Verification items for the finished model (mm, model axes). Give positions to 0.01 mm unless a question says otherwise; leave off trailing zeros. Loops run counter-clockwise (first coordinate to the right, second up) from the corner with the lowest first, then second, coordinate; pieces in that order, holes last. Notation, with made-up numbers: (-28, 11) - (-3, 11) arc R22 cw to (-3, 39) - close; hole circle Ø8 at (-28, -0.5). An arc over 180 degrees is marked (long way). Answer in a Markdown table with one row per item.
```python
from build123d import *

# Parameters (mm, degrees)
SKETCH1_R             = 2.625
BOSS_EXTRUDE1_DEPTH   = 4
FILLET1_R             = 35
FILLET2_R             = 8
SKETCH2_R             = 5.05
CUT_EXTRUDE1_DEPTH    = 1
FILLET3_R             = 1
FILLET7_R             = 4
MIRROR1_OUTLINE_R     = 5.05
MIRROR1_DEPTH         = 4
MIRROR1_2_OUTLINE_R   = 5.05
MIRROR1_2_OUTLINE_R_2 = 2.625
MIRROR1_2_DEPTH       = 3
FILLET6_R             = 1
SKETCH3_R             = 6
BOSS_EXTRUDE2_DEPTH   = 4
FILLET8_R             = 4


with BuildPart() as part:
    # Sketch1 → Boss-Extrude1 (new body)
    with BuildSketch(Plane(origin=(0, 0, 0), x_dir=(1, 0, 0), z_dir=(0, 1, 0))):
        with BuildLine():
            Line((-0.828427125, -40), (15.171572875, -40))
            ThreePointArc((15.171572875, -40), (16.585786438, -39.414213562), (17.171572875, -38))
            Line((17.171572875, -38), (17.171572875, -10.175438596))
            Line((17.171572875, -10.175438596), (17.171572875, 18))
            ThreePointArc((17.171572875, 18), (16.585786438, 19.414213562), (15.171572875, 20))
            Line((15.171572875, 20), (-40.828427125, 20))
            ThreePointArc((-40.828427125, 20), (-42.242640687, 19.414213562), (-42.828427125, 18))
            Line((-42.828427125, 18), (-42.828427125, 2))
            Line((-42.828427125, 2), (-42.828427125, -4))
            Line((-42.828427125, -4), (-6.828427125, -40))
            Line((-6.828427125, -40), (-0.828427125, -40))
        make_face()
        with Locations(Location((-32.828427125, 10, 0), (0, 0, 270))):
            Circle(SKETCH1_R, mode=Mode.SUBTRACT)
        with Locations(Location((-12.828427125, 10, 0), (0, 0, 270))):
            Circle(SKETCH1_R, mode=Mode.SUBTRACT)
        with Locations(Location((7.171572875, -32, 0), (0, 0, 270))):
            Circle(SKETCH1_R, mode=Mode.SUBTRACT)
        with Locations(Location((7.171572875, 10, 0), (0, 0, 270))):
            Circle(SKETCH1_R, mode=Mode.SUBTRACT)
        with Locations(Location((7.171572875, -11, 0), (0, 0, 270))):
            Circle(SKETCH1_R, mode=Mode.SUBTRACT)
        Polygon((0, 0), (0, -34.343145751), (-4, -34.343145751), (-34.343145751, -4), (-34.343145751, 0), align=None, mode=Mode.SUBTRACT)
    extrude(amount=BOSS_EXTRUDE1_DEPTH)

    # Fillet1
    # the kernel refuses this fillet: 35 mm, written as the material it adds along each edge
    with BuildSketch(Plane(origin=(0, 0, 0), x_dir=(-1, 0, 0), z_dir=(0, 1, 0))) as fillet1_piece_1:
        with BuildLine():
            CenterArc((34.993835779, 35), FILLET1_R, 181.075348167, 88.924651833)
            Line((0, 34.343145751), (-0.699876716, 34.330008666))
            ThreePointArc((-0.699876716, 34.330008666), (-0.7, 17.171572875), (-0.7, 0))
            Line((-0.7, 0), (0, -0.7))
            Line((0, -0.7), (34.993835779, -0.7))
            Line((34.993835779, -0.7), (34.993835779, 0))
        make_face()
    extrude(amount=4)

    # Fillet2
    # the kernel refuses this fillet: 8 mm, written as the material it adds along each edge
    with BuildSketch(Plane(origin=(0, 0, 34.343145751), x_dir=(-0.13953759415061998, 0, -0.9902167741553647), z_dir=(0, 1, 0))) as fillet2_piece_1:
        with BuildLine():
            CenterArc((7.497620247, 7.941288924), FILLET2_R, 209.838221464, 67.107520075)
            Line((0.558150377, 3.960867097), (0, 0))
            ThreePointArc((0, 0), (4.232527559, -0.256860958), (8.465055117, 0))
        make_face()
    extrude(amount=4)
    with BuildSketch(Plane(origin=(-34.343145751, 4, 0.006049059), x_dir=(0.9902532983948017, 0, 0.13927815700322774), z_dir=(0, -1, 0))) as fillet2_piece_2:
        with BuildLine():
            CenterArc((7.49233694, 7.941371943), FILLET2_R, 209.887169965, 67.053653065)
            Line((0.556270126, 3.955023093), (0, 0))
            ThreePointArc((0, 0), (4.229545047, -0.256497749), (8.459090094, 0))
        make_face()
    extrude(amount=4)
    # the kernel refuses this fillet: 8 mm, written as the material it takes off along each edge
    with BuildSketch(Plane(origin=(-42.828427125, -8.284271247, 4), x_dir=(0.7071067811865472, 0, 0.7071067811865477), z_dir=(0, 1, 0)), Plane(origin=(-6.828427125, -8.284271247, 40), x_dir=(1, 0, 0), z_dir=(0, 1, 0))) as fillet2_2_piece_1:
        with BuildLine():
            CenterArc((FILLET2_R * 0.414213562373, FILLET2_R), FILLET2_R, 225, 45)
            Line((-FILLET2_R * 0.292893218813, FILLET2_R * 0.292893218813), (0, 0))
            Line((0, 0), (FILLET2_R * 0.414213562373, 0))
        make_face()
    extrude(amount=20.568542495, mode=Mode.SUBTRACT)

    # Sketch2 → Cut-Extrude1 (cut)
    with BuildSketch(Plane(origin=(0, 4, 0), x_dir=(1, 0, 0), z_dir=(0, 1, 0))):
        with Locations(Location((-32.828427125, 10, 0), (0, 0, 270))):
            Circle(SKETCH2_R)
        with Locations(Location((-12.828427125, 10, 0), (0, 0, 270))):
            Circle(SKETCH2_R)
        with Locations(Location((7.171572875, 10, 0), (0, 0, 270))):
            Circle(SKETCH2_R)
        with Locations(Location((7.171572875, -11, 0), (0, 0, 270))):
            Circle(SKETCH2_R)
        with Locations(Location((7.171572875, -32, 0), (0, 0, 270))):
            Circle(SKETCH2_R)
    extrude(amount=-CUT_EXTRUDE1_DEPTH, mode=Mode.SUBTRACT)

    # Fillet3
    fillet3_edges = [part.edges().sort_by_distance(p)[0] for p in [
        (-12.828427125, 4, -20),
        (-42.242640687, 4, -19.414213562),
        (-42.828427125, 4, -8.656854249),
        (16.585786438, 4, 39.414213562),
        (17.171572875, 4, 10),
        (-24.828427125, 4, 22),
        (5.828427125, 4, 40),
        (-6.576186085, 4, 39.39103626),
        (-42.219463385, 4, 3.74775896),
        (16.585786438, 4, -19.414213562),
    ]]
    fillet(fillet3_edges, radius=FILLET3_R)

    # Fillet7
    fillet7_edges = [part.edges().sort_by_distance(p)[0] for p in [
        (-34.343145751, 2, 4),
        (-4, 2, 34.343145751),
    ]]
    fillet(fillet7_edges, radius=FILLET7_R)

    # Mirror1: read off the stored shape, not the designer's step
    # Mirror1 outline → Mirror1 (add)
    with BuildSketch(Plane(origin=(0, 0, 0), x_dir=(1, 0, 0), z_dir=(0, 1, 0))):
        with BuildLine():
            ThreePointArc((-3.514718626, 60), (-6.576186085, 59.39103626), (-9.171572875, 57.656854249))
            Line((-9.171572875, 57.656854249), (-40.485281374, 26.343145751))
            ThreePointArc((-40.485281374, 26.343145751), (-42.219463385, 23.74775896), (-42.828427125, 20.686291501))
            Line((-42.828427125, 20.686291501), (-42.828427125, 2))
            ThreePointArc((-42.828427125, 2), (-42.560477932, 1), (-41.828427125, 0.267949192))
            Line((-41.828427125, 0.267949192), (-41.828427125, -0.686291501))
            ThreePointArc((-41.828427125, -0.686291501), (-41.295583852, -3.365075528), (-39.778174593, -5.636038969))
            Line((-39.778174593, -5.636038969), (-8.464466094, -36.949747468))
            ThreePointArc((-8.464466094, -36.949747468), (-6.193502652, -38.467156728), (-3.514718626, -39))
            Line((-3.514718626, -39), (15.171572875, -39))
            ThreePointArc((15.171572875, -39), (15.878679656, -38.707106781), (16.171572875, -38))
            Line((16.171572875, -38), (16.171572875, 0.267949192))
            ThreePointArc((16.171572875, 0.267949192), (16.903623683, 1), (17.171572875, 2))
            Line((17.171572875, 2), (17.171572875, 58))
            ThreePointArc((17.171572875, 58), (16.585786438, 59.414213562), (15.171572875, 60))
            Line((15.171572875, 60), (-3.514718626, 60))
        make_face()
        with BuildLine():
            ThreePointArc((-0.926569244, -27.509231599), (-3.268603973, -31.412129037), (-7.746610443, -30.596535308))
            Line((-7.746610443, -30.596535308), (-30.592327017, -7.750818734))
            ThreePointArc((-30.592327017, -7.750818734), (-31.406448507, -3.269563854), (-27.497905753, -0.931245518))
            ThreePointArc((-27.497905753, -0.931245518), (-26.72605518, -1.020502526), (-25.966503884, -1.184215537))
            ThreePointArc((-25.966503884, -1.184215537), (-10.249403108, -10.246958736), (-1.181193425, -25.960906179))
            ThreePointArc((-1.181193425, -25.960906179), (-1.015828492, -26.728811048), (-0.926569244, -27.509231599))
        make_face(mode=Mode.SUBTRACT)
        with Locations((-32.828427125, 10)):
            Circle(MIRROR1_OUTLINE_R, mode=Mode.SUBTRACT)
        with Locations((7.171572875, -32)):
            Circle(MIRROR1_OUTLINE_R, mode=Mode.SUBTRACT)
        with Locations((-12.828427125, 10)):
            Circle(MIRROR1_OUTLINE_R, mode=Mode.SUBTRACT)
        with Locations((7.171572875, -11)):
            Circle(MIRROR1_OUTLINE_R, mode=Mode.SUBTRACT)
        with Locations((7.171572875, 10)):
            Circle(MIRROR1_OUTLINE_R, mode=Mode.SUBTRACT)
        with BuildLine():
            ThreePointArc((-25.960906179, 21.181193425), (-30.576929417, 21.327068181), (-34.343145751, 24))
            Line((-34.343145751, 24), (-4, 54.343145751))
            ThreePointArc((-4, 54.343145751), (-1.330496844, 50.57891176), (-1.184215537, 45.966503884))
            ThreePointArc((-1.184215537, 45.966503884), (-10.246958736, 30.249403108), (-25.960906179, 21.181193425))
        make_face(mode=Mode.SUBTRACT)
        with Locations((7.171572875, 31)):
            Circle(MIRROR1_OUTLINE_R, mode=Mode.SUBTRACT)
        with Locations((7.171572875, 52)):
            Circle(MIRROR1_OUTLINE_R, mode=Mode.SUBTRACT)
    extrude(amount=MIRROR1_DEPTH)

    # Mirror1 2 outline → Mirror1 2 (add)
    # profile 1 of 2: a face of its own
    with BuildSketch(Plane(origin=(0, 0, 0), x_dir=(1, 0, 0), z_dir=(0, 1, 0))):
        with Locations((7.171572875, 31)):
            Circle(MIRROR1_2_OUTLINE_R)
        with Locations((7.171572875, 31)):
            Circle(MIRROR1_2_OUTLINE_R_2, mode=Mode.SUBTRACT)
    # profile 2 of 2: a face of its own
    with BuildSketch(Plane(origin=(0, 0, 0), x_dir=(1, 0, 0), z_dir=(0, 1, 0))):
        with Locations((7.171572875, 52)):
            Circle(MIRROR1_2_OUTLINE_R)
        with Locations((7.171572875, 52)):
            Circle(MIRROR1_2_OUTLINE_R_2, mode=Mode.SUBTRACT)
    extrude(amount=MIRROR1_2_DEPTH)

    # Fillet6
    fillet6_edges = [part.edges().sort_by_distance(p)[0] for p in [
        (-42.828427125, 4, -11.34314575),
        (-42.219463385, 4, -23.74775896),
        (-24.828427125, 4, -42),
        (-6.576186085, 4, -59.39103626),
        (5.828427125, 4, -60),
        (16.585786438, 4, -59.414213563),
        (17.171572875, 4, -30),
    ]]
    fillet(fillet6_edges, radius=FILLET6_R - 0.0001)  # a hair under: the kernel refuses the full size

    # Sketch3 → Boss-Extrude2 (add)
    with BuildSketch(Plane(origin=(0, 4, 0), x_dir=(1, 0, 0), z_dir=(0, 1, 0))):
        with Locations((7.171572875, 10)):
            Circle(SKETCH3_R)
    extrude(amount=-BOSS_EXTRUDE2_DEPTH)

    # Fillet8
    fillet8_edges = [part.edges().sort_by_distance(p)[0] for p in [
        (-4, 2, -54.343145751),
        (-34.343145751, 2, -24),
    ]]
    fillet(fillet8_edges, radius=FILLET8_R)


solid = part.part
```
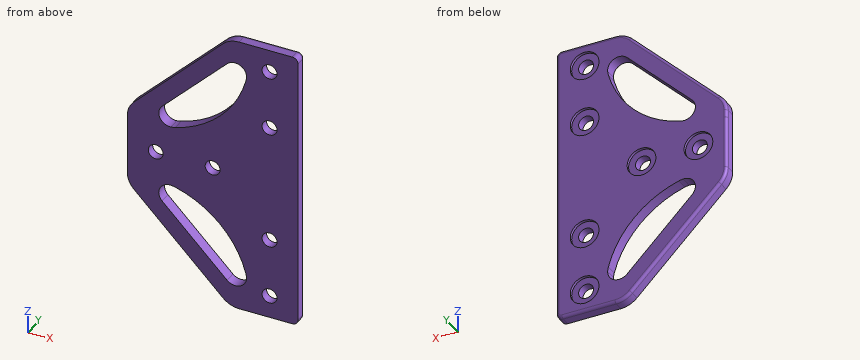
Q1. Thickness scan on line 1 (X direction, y = 3.85, z = -8.5); line 2 (X direction, y = 3.2, z = 11); line 3 (Z direction, x = -8, y = 2.8). Record the ranges inside material, lowest first.
Completed:
| item | result |
|---|---|
| line 1 | -42.36 to -37.65, -28.01 to -17.65, -8.01 to 16.7 |
| line 2 | -35.8 to -27.34, -9.52 to 2.12, 12.22 to 17.15 |
| line 3 | -58.62 to -50.34, -32.72 to 12.72, 30.34 to 38.62 |
Q2. Sectioned sample at B-B (y = 1.15). Give the number of separate pieces and of enclosed holes in the cut face, and give its area (3 significant figures).
Completed:
| item | result |
|---|---|
| separate pieces | 1 |
| enclosed holes | 8 |
| area | 3,730 mm^2 |
Q3. Sectioned sample at A-A (z = -10). Record the cut outline in (x, y), and give its area (3 significant figures).
Completed:
| item | result |
|---|---|
| outline | (-42.83, 0) - (-35.45, 0) - (-35.45, 3) - (-37.88, 3) - (-37.88, 4) - (-41.83, 4) arc R1 ccw to (-42.83, 3) - close; (-30.2, 0) - (-15.45, 0) - (-15.45, 3) - (-17.88, 3) - (-17.88, 4) - (-27.78, 4) - (-27.78, 3) - (-30.2, 3) - close; (-10.2, 0) - (17.17, 0) - (17.17, 3) arc R1 ccw to (16.17, 4) - (-7.78, 4) - (-7.78, 3) - (-10.2, 3) - close |
| area | 188 mm^2 |
Q4. Go/stop test with a flat-tipped pin: P1, Ø7, axis at x = 7.17, z = -52, coming from the +Y side. Record where the tip stops, or that it passes through.
Completed:
| item | result |
|---|---|
| P1 | y = 3 |
